```python
from build123d import *

# Parameters (mm, degrees)
F1_DEPTH  = 18.034
F2_R      = 6.0450244322
F2_R_2    = 6.2773017577
F3_DEPTH  = 11.938
F4_W      = 18.034
F4_H      = 12.7806511284
F5_DEPTH  = 4.572
F7_DEPTH  = 6.096
F8_W      = 18.034
F8_H      = 41.8857587501
F9_DEPTH  = 2.286
F10_W     = 5.6385421194
F10_H     = 6.2931925058
F11_DEPTH = 9.652
F12_W     = 5.6385421194
F12_H     = 4.826
F13_DEPTH = 5.334


with BuildPart() as f1:
    # F0 (on Right) → F1 (new body)
    with BuildSketch(Plane.YZ):
        Polygon((39.2854847014, 32.0903435349), (-41.3001254201, 32.0903435349), (-62.0221421123, 17.1244423836), (-41.3001254201, 0), (39.2854847014, 0), align=None)
    extrude(amount=F1_DEPTH)

    # F2 (on face) → F3 (cut)
    with BuildSketch(Plane(origin=(0, 39.2854847014, 0), x_dir=(-1, 0, 0), z_dir=(0, 1, 0))):
        with Locations((-9.5175812021, 23.9161904901)):
            Circle(F2_R)
        with Locations((-9.0148737654, 9.5570040867)):
            Circle(F2_R_2)
    extrude(amount=-F3_DEPTH, mode=Mode.SUBTRACT)

    # F4 (on face) → F5 (cut)
    with BuildSketch(Plane(origin=(0, -29.3891718919, 40.6926989799), x_dir=(1, 0, 0), z_dir=(0, -0.5854905592, 0.8106792246))):
        with Locations((9.017, -21.0828860338)):
            Rectangle(F4_W, F4_H)
    extrude(amount=-F5_DEPTH, mode=Mode.SUBTRACT)

    # F6 (on face) → F7 (cut)
    with BuildSketch(Plane(origin=(0, 0, 0), x_dir=(1, 0, 0), z_dir=(0, 0, -1))):
        Polygon((4.0432531387, 26.875609532), (4.0432531387, -24.9088313431), (14.6540477872, -24.865726009), (14.6540477872, 26.875609532), align=None)
    extrude(amount=-F7_DEPTH, mode=Mode.SUBTRACT)

    # F8 (on face) → F9 (cut)
    with BuildSketch(Plane.XY.offset(32.0903435349)):
        with Locations((9.017, 5.4818768986)):
            Rectangle(F8_W, F8_H)
    extrude(amount=-F9_DEPTH, mode=Mode.SUBTRACT)

    # F10 (on face) → F11 (join)
    with BuildSketch(Plane.XY.offset(29.8043435349)):
        with Locations((9.5915335696, 17.6502466202)):
            Rectangle(F10_W, F10_H)
    extrude(amount=F11_DEPTH)

    # F12 (on face) → F13 (join)
    with BuildSketch(Plane.XZ.offset(-14.5036503673)):
        with Locations((9.5915335696, 32.2173435349)):
            Rectangle(F12_W, F12_H)
    extrude(amount=F13_DEPTH)


solid = f1.part
```
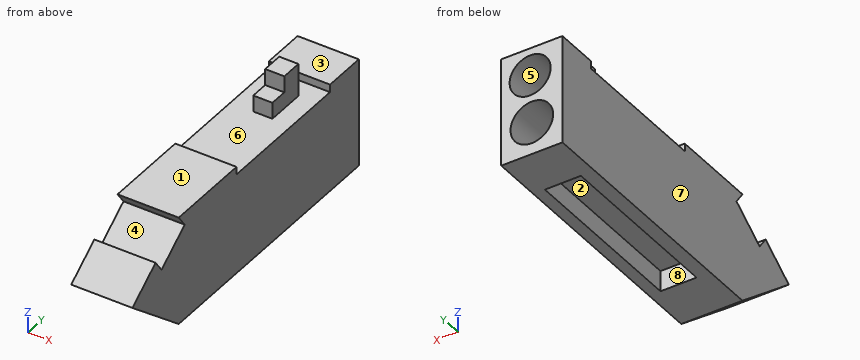
Geometry: final body of the model. Coordinates: model frame, mm. Face numbers are marked on the shaded views. A direction names the side the tool comes from. Coordinates: 2 decimals unless noted, no trailing zeros. Order: outer loops, then holes, each group sorted by start corner. A loop starts at its lowest first (then second) coordinate and runs counter-clockwise, first axis right, second up. Notation, with made-up numbers: (-26.5, 27) -> (25.5, 27) arc R17 cw to (25.5, 44) -> close; hole circle Ø2 at (-37.5, 46.25). An arc over 180 degrees is marked (long way). Answer in a Markdown table with one row per item.
Item 1: Section D-D on y = 18.5. Output: boundary loops of the cut face in (x, z).
Return value:
| item | result |
|---|---|
| outline | (0, 0) -> (4.04, 0) -> (4.04, 6.1) -> (14.65, 6.1) -> (14.65, 0) -> (18.03, 0) -> (18.03, 29.8) -> (12.41, 29.8) -> (12.41, 39.46) -> (6.77, 39.46) -> (6.77, 29.8) -> (0, 29.8) -> close |
Item 2: Section C-C on z = 27.5. Output: boundary loops of the cut face in (x, y).
Return value:
| item | result |
|---|---|
| outline | (0, -39.85) -> (18.03, -39.85) -> (18.03, 39.29) -> (14.39, 39.29) -> (14.39, 27.35) -> (4.65, 27.35) -> (4.65, 39.29) -> (0, 39.29) -> close |
Item 3: Section A-A on y = -20.5. Output: boundary loops of the cut face in (x, z).
Return value:
| item | result |
|---|---|
| outline | (0, 0) -> (4.04, 0) -> (4.04, 6.1) -> (14.65, 6.1) -> (14.65, 0) -> (18.03, 0) -> (18.03, 32.09) -> (0, 32.09) -> close |
Item 4: Ray query, L1, parallel to X at y = 0.5, z = 6; L2, parallel to Z at x = 6.5, y = 32; L3, parallel to Y at x = 9, z = 30.5. Return the intervals inside material, ascending.
Return value:
| item | result |
|---|---|
| L1 | x = 0 to 4.04, 14.65 to 18.03 |
| L2 | z = 0 to 3.81, 15.31 to 18.68, 29.15 to 32.09 |
| L3 | y = -40.15 to -15.46, 9.17 to 20.8, 26.42 to 39.29 |
Item 5: Access query for the marked faces 1, 2, 3, 4 and 5. Directions: +Z, -Z, +X, -X, +Y, -Y. A direction counts if a zero-diameter tool reaches every point of the face in a straight line with its end or side. Return the directions, or none.
Return value:
| item | result |
|---|---|
| face 1 | +Z, +X, -X, -Y |
| face 2 | -Z |
| face 3 | +Z, +X, -X, +Y |
| face 4 | +X, -X |
| face 5 | +Y |
Item 6: Section B-B on x = 17. Output: boundary loops of the cut face in (y, z), plus the area to 3 significant figures.
Return value:
| item | result |
|---|---|
| outline | (-62.02, 17.12) -> (-41.3, 0) -> (39.29, 0) -> (39.29, 32.09) -> (26.42, 32.09) -> (26.42, 29.8) -> (-15.46, 29.8) -> (-15.46, 32.09) -> (-41.3, 32.09) -> (-38.62, 28.38) -> (-48.98, 20.9) -> (-51.66, 24.61) -> close |
| area | 2,760 mm² |
Item 7: Contact query for flat-ended pins moving along their axis: P1, Ø5.5, axis at x = 5, y = 8, coming from the +Z side; P2, Ø2, axis at x = 5.5, y = 15.5, coming from the +Z side; P3, Ø12, axis at y = -49.5, z = 34, coming from the +X side; P4, Ø7.5, axis at y = 17, z = 36.5, coming from the -X side. Output: stop coordinate, or through.
Return value:
| item | result |
|---|---|
| P1 | stops at z = 34.63 |
| P2 | stops at z = 29.8 |
| P3 | passes through |
| P4 | stops at x = 6.77 |
Item 8: Draft query along X for the marked faces 6, 7 and 8. Return one class per face: released by +X, released by -X, zero draft, split by the parting line, or undercut.
Return value:
| item | result |
|---|---|
| face 6 | zero draft |
| face 7 | released by -X |
| face 8 | undercut |
